Check sheet for the modelled part. Datum: model origin and axes. Units: mm. A direction names the side the tool comes from. Coordinates: 2 decimals unless noted, no trailing zeros. Loops run counter-clockwise (first coordinate to the right, second up) from the corner with the lowest first, then second, coordinate; pieces in that order, holes last. Notation, with made-up numbers: (74, 23.5) - (97, 23.5) arc R29 cw to (97, 47.5) - close; hole circle Ø9 at (58, 13). An arc over 180 degrees is marked (long way). Answer as a JSON object with one key per item and string values. Group by question number.
from build123d import *

# Parameters (mm, degrees)
SHELL1_T  = -1
FILLET1_R = 1
FILLET2_R = 1


with BuildPart() as part:
    # Sketch1 → Revolve1 (revolve)
    with BuildSketch(Plane.XY):
        Polygon((0, 0), (0, 30), (-7.5, 30), (-7.5, 25), (-10, 25), (-10, 0), align=None)
    revolve(axis=Axis((0, 30, 0), (0, 1, 0)))

    # Shell1
    shell1_openings = [part.faces().sort_by_distance(p)[0] for p in [
        (0, 30, -7.5),
    ]]
    offset(amount=SHELL1_T, openings=shell1_openings, kind=Kind.INTERSECTION)

    # Fillet1
    fillet1_edges = [part.edges().sort_by_distance(p)[0] for p in [
        (7.5, 25, 0),
        (10, 25, 0),
        (10, 0, 0),
    ]]
    fillet(fillet1_edges, radius=FILLET1_R)

    # Fillet2
    fillet2_edges = [part.edges().sort_by_distance(p)[0] for p in [
        (6.5, 24, 0),
    ]]
    fillet(fillet2_edges, radius=FILLET2_R)


solid = part.part
1. Sectioned sample at B-B on y = 2.5. Record the cut outline in (x, z).
2. Sectioned sample at A-A on z = 0. Record the cut outline in (x, y).
3. Release check for a two-part mould opening along Z. For faces 1 (the face through (-6, 30, 3)), 2 (the face through (0, 1, 0)), 3 (the face through (7.493, 27.972, 0.33)) record: released by +Z, released by -Z, zero draft, split by the parting line, or undercut.
4. Sectioned sample at C-C on x = 0. Record the cut outline in (y, z).
5. Material ranges on line 1 (Z direction, x = 0, y = 27.9); line 2 (Z direction, x = 0, y = 18.75); line 3 (Y direction, x = 5, z = -6.75) (3 decimals), recorded low to high.
6. Access from +Z, -Z, +X, -X, +Y, -Y to the whole of each face (thin tool, end or side, straight path). Record for faces 4 (the face through (2.17, 12.34, -9.76)), 5 (the face through (5.158, 27.465, -3.955)), 6 (the face through (1.172, 12.339, 8.923)).
7. Gauge pin test, flat ends, axial feed: pin 1 (4 mm diameter, centred on x = -4, z = 2.5, fed in from -Y); pin 2 (10 mm diameter, centred on y = 16.5, z = -6, fed in from -X); pin 3 (1 mm diameter, centred on x = -2, y = 23.5, fed in from -Z); pin 4 (9 mm diameter, centred on x = 0.5, z = 0, fed in from +Y). Record the tip position at first contact, or that the pin passes through.
Answers follow:
{
 "1": {"outline": "circle Ø20 at (0, 0); hole circle Ø18 at (0, 0)"},
 "2": {"outline": "(-10, 1) arc R1 ccw to (-9, 0) - (9, 0) arc R1 ccw to (10, 1) - (10, 24) arc R1 ccw to (9, 25) - (8.5, 25) arc R1 cw to (7.5, 26) - (7.5, 30) - (6.5, 30) - (6.5, 25) arc R1 ccw to (7.5, 24) - (9, 24) - (9, 1) - (-9, 1) - (-9, 24) - (-7.5, 24) arc R1 ccw to (-6.5, 25) - (-6.5, 30) - (-7.5, 30) - (-7.5, 26) arc R1 cw to (-8.5, 25) - (-9, 25) arc R1 ccw to (-10, 24) - close"},
 "3": {"face 1": "zero draft", "face 2": "undercut", "face 3": "split by the parting line"},
 "4": {"outline": "(0, -9) arc R1 ccw to (1, -10) - (24, -10) arc R1 ccw to (25, -9) - (25, -8.5) arc R1 cw to (26, -7.5) - (30, -7.5) - (30, -6.5) - (25, -6.5) arc R1 ccw to (24, -7.5) - (24, -9) - (1, -9) - (1, 9) - (24, 9) - (24, 7.5) arc R1 ccw to (25, 6.5) - (30, 6.5) - (30, 7.5) - (26, 7.5) arc R1 cw to (25, 8.5) - (25, 9) arc R1 ccw to (24, 10) - (1, 10) arc R1 ccw to (0, 9) - close"},
 "5": {"line 1": "z = -7.5 to -6.5, 6.5 to 7.5", "line 2": "z = -10 to -9, 9 to 10", "line 3": "y = 0 to 1, 24 to 25.005"},
 "6": {"face 4": "+Y, -Y", "face 5": "+Y", "face 6": "none"},
 "7": {"pin 1": "stops at y = 0", "pin 2": "stops at x = -9.95", "pin 3": "stops at z = -9.89", "pin 4": "stops at y = 1"}
}
